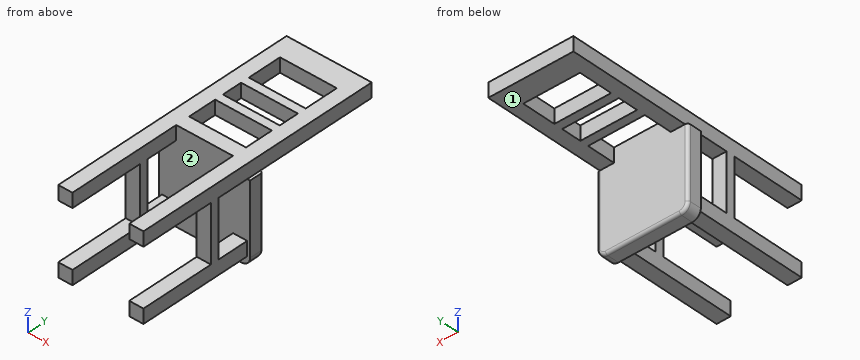
```python
from build123d import *

# Parameters (mm, degrees)
SKETCH1_W             = 5
SKETCH1_H             = 5
BOSS_EXTRUDE1_DEPTH   = 40
BOSS_EXTRUDE1_2_DEPTH = 40
BOSS_EXTRUDE1_3_DEPTH = 40
BOSS_EXTRUDE1_4_DEPTH = 40
BOSS_EXTRUDE2_DEPTH   = 5
SKETCH3_W             = 5
SKETCH3_H             = 5
BOSS_EXTRUDE3_DEPTH   = 40
SKETCH4_W             = 30
SKETCH4_H             = 5
BOSS_EXTRUDE4_DEPTH   = 8
SKETCH5_W             = 5
SKETCH5_H             = 3
BOSS_EXTRUDE5_DEPTH   = 20
SKETCH6_W             = 5
SKETCH6_H             = 3
BOSS_EXTRUDE6_DEPTH   = 20
FILLET1_R             = 3
FILLET2_R             = 1


with BuildPart() as part:
    # Sketch1 → Boss-Extrude1 (new body)
    with BuildSketch(Plane(origin=(0, 0, 0), x_dir=(1, 0, 0), z_dir=(0, 1, 0))):
        with Locations((-27.5, 2.5)):
            Rectangle(SKETCH1_W, SKETCH1_H)
    extrude(amount=BOSS_EXTRUDE1_DEPTH)



with BuildPart() as body_2:
    # Sketch1 → Boss-Extrude1 2 (new body)
    with BuildSketch(Plane(origin=(0, 0, 0), x_dir=(1, 0, 0), z_dir=(0, 1, 0))):
        with Locations((-2.5, 2.5)):
            Rectangle(SKETCH1_W, SKETCH1_H)
    extrude(amount=BOSS_EXTRUDE1_2_DEPTH)


with BuildPart() as body_3:
    # Sketch1 → Boss-Extrude1 3 (new body)
    with BuildSketch(Plane(origin=(0, 0, 0), x_dir=(1, 0, 0), z_dir=(0, 1, 0))):
        with Locations((-2.5, 27.5)):
            Rectangle(SKETCH1_W, SKETCH1_H)
    extrude(amount=BOSS_EXTRUDE1_3_DEPTH)



with BuildPart() as body_4:
    # Sketch1 → Boss-Extrude1 4 (new body)
    with BuildSketch(Plane(origin=(0, 0, 0), x_dir=(1, 0, 0), z_dir=(0, 1, 0))):
        with Locations((-27.5, 27.5)):
            Rectangle(SKETCH1_W, SKETCH1_H)
    extrude(amount=BOSS_EXTRUDE1_4_DEPTH)


with BuildPart() as body_3_1:
    add(body_3.part)

    add(body_4.part)  # Boss-Extrude2 merges body 4
    # Sketch2 → Boss-Extrude2 (add)
    with BuildSketch(Plane(origin=(0, 40, 0), x_dir=(1, 0, 0), z_dir=(0, 1, 0))):
        Polygon((-5, 0), (-5, 5), (1, 5), (1, 33), (-31, 33), (-31, 5), (-30, 5), (-25, 5), (-25, 0), align=None)
    extrude(amount=BOSS_EXTRUDE2_DEPTH)


with BuildPart() as part_1:
    add(part.part)

    add(body_2.part)  # Boss-Extrude3 merges body 2

    add(body_3_1.part)  # Boss-Extrude3 merges body 3
    # Sketch3 → Boss-Extrude3 (add)
    with BuildSketch(Plane(origin=(0, 40, 0), x_dir=(1, 0, 0), z_dir=(0, 1, 0))):
        with Locations((-27.5, 2.5)):
            Rectangle(SKETCH3_W, SKETCH3_H)
        with Locations((-2.5, 2.5)):
            Rectangle(SKETCH3_W, SKETCH3_H)
    extrude(amount=BOSS_EXTRUDE3_DEPTH)

    # Sketch4 → Boss-Extrude4 (add)
    with BuildSketch(Plane(origin=(0, 80, 0), x_dir=(1, 0, 0), z_dir=(0, 1, 0))):
        with Locations((-15, 2.5)):
            Rectangle(SKETCH4_W, SKETCH4_H)
    extrude(amount=BOSS_EXTRUDE4_DEPTH)

    # Sketch5 → Boss-Extrude5 (add)
    with BuildSketch(Plane(origin=(-25, 0, 0), x_dir=(0, 0, -1), z_dir=(1, 0, 0))):
        with Locations((2.5, 66.5)):
            Rectangle(SKETCH5_W, SKETCH5_H)
        with Locations((2.5, 56.5)):
            Rectangle(SKETCH5_W, SKETCH5_H)
    extrude(amount=BOSS_EXTRUDE5_DEPTH)

    # Sketch6 → Boss-Extrude6 (add)
    with BuildSketch(Plane(origin=(0, 0, -5), x_dir=(-1, 0, 0), z_dir=(0, 0, -1))):
        with Locations((2.5, 27.5)):
            Rectangle(SKETCH6_W, SKETCH6_H)
        with Locations((27.5, 27.5)):
            Rectangle(SKETCH6_W, SKETCH6_H)
    extrude(amount=BOSS_EXTRUDE6_DEPTH)

    # Fillet1
    fillet1_edges = [part_1.edges().sort_by_distance(p)[0] for p in [
        (1, 42.5, -33),
        (-31, 42.5, -33),
    ]]
    fillet(fillet1_edges, radius=FILLET1_R)

    # Fillet2
    fillet2_edges = [part_1.edges().sort_by_distance(p)[0] for p in [
        (-31, 45, -17.5),
        (-30.121320344, 45, -32.121320344),
        (-15, 45, -33),
        (0.121320344, 45, -32.121320344),
        (1, 45, -17.5),
    ]]
    fillet(fillet2_edges, radius=FILLET2_R)


solid = part_1.part
```
Here's how the part is built. I have some questions about the finished solid (model axes, mm). Face numbers are marked on the shaded views. Give positions to 0.01 mm unless a question says otherwise; leave off trailing zeros. Write each loop counter-clockwise with the first axis right and the second up, starting at its lowest first coordinate (ties: lowest second). Pieces come first, ordered by that corner, then holes. Notation, with made-up numbers: (9.5, 17.25) -> (45.5, 17.25) arc R26 ccw to (45.5, 31.25) -> close; hole circle Ø8 at (-32.5, 50). An arc over 180 degrees is marked (long way). Use one line per item in the form item = value.
1) I'm going to push flat-ended pins straight in: pin 1 (1.5 mm diameter, centred on x = -2.5, z = -10, fed in from -Y); pin 2 (5.5 mm diameter, centred on x = -27, y = 35.5, fed in from -Z); pin 3 (2 mm diameter, centred on y = 57.5, z = -3.5, fed in from -X). Where does each tip first touch, or does it pass through?
Verdict:
pin_1 = 26
pin_2 = -30
pin_3 = -30
2) Suppose I cut it at B-B (y = 46). Please give me the cut outline in (x, z).
Verdict:
outline = (-30, -5) -> (-25, -5) -> (-25, 0) -> (-30, 0) -> close; (-5, -5) -> (0, -5) -> (0, 0) -> (-5, 0) -> close
3) We'd pull the mould along Y, two halves only. Please class the marked faces 1 and 2: +Y half, -Y half, draft (parallel to the pull), parting line (faces both ways), or undercut.
Verdict:
face_1 = draft
face_2 = undercut
4) Suppose I cut it at D-D (z = -2). Please give me the cut outline in (x, y).
Verdict:
outline = (-30, 0) -> (-25, 0) -> (-25, 40) -> (-5, 40) -> (-5, 0) -> (0, 0) -> (0, 88) -> (-30, 88) -> close; hole (-25, 45) -> (-5, 45) -> (-5, 55) -> (-25, 55) -> close; hole (-25, 58) -> (-5, 58) -> (-5, 65) -> (-25, 65) -> close; hole (-25, 68) -> (-5, 68) -> (-5, 80) -> (-25, 80) -> close
5) Suppose I cut it at C-C (x = -12.5). Please give me the cut outline in (y, z), and give its area (3 significant figures).
Verdict:
outline = (40, -33) -> (44, -33) arc R1 ccw to (45, -32) -> (45, 0) -> (40, 0) -> close; (55, -5) -> (58, -5) -> (58, 0) -> (55, 0) -> close; (65, -5) -> (68, -5) -> (68, 0) -> (65, 0) -> close; (80, -5) -> (88, -5) -> (88, 0) -> (80, 0) -> close
area = 235 mm2
6) If I drill on L1, parallel to Y at x = -15, z = -3.5; L2, parallel to Y at x = -2, z = -12; L3, parallel to Z at x = -28.5, y = 32, over which ranges is the centre line in solid material (lowest first)? Write a range as [from, to].
Verdict:
L1 = [40, 45], [55, 58], [65, 68], [80, 88]
L2 = [26, 29], [40, 45]
L3 = [-30, -25], [-5, 0]
7) Suppose I cut it at A-A (z = -18.5). Please give me the cut outline in (x, y), and give its area (3 significant figures).
Verdict:
outline = (-31, 40) -> (1, 40) -> (1, 44) arc R1 ccw to (0, 45) -> (-30, 45) arc R1 ccw to (-31, 44) -> close; (-30, 26) -> (-25, 26) -> (-25, 29) -> (-30, 29) -> close; (-5, 26) -> (0, 26) -> (0, 29) -> (-5, 29) -> close
area = 190 mm2
